Autodesk Inventor part; units mm, degrees
ref_plane "YZ Plane" through (0, 0, 0) normal (1, 0, 0) x (0, 1, 0)
ref_plane "XZ Plane" through (0, 0, 0) normal (0, 1, 0) x (-1, 0, 0)
ref_plane "XY Plane" through (0, 0, 0) normal (0, 0, 1) x (1, 0, 0)
sketch "Sketch1" plane through (0, 0, 0) normal (0, 0, 1) x (1, 0, 0)
  line L0 (0, 0) -> (50.8, 0)
  line L1 (50.8, 0) -> (50.8, 50.8)
  line L2 (50.8, 50.8) -> (0, 50.8)
  line L3 (0, 50.8) -> (0, 0)
  line L4 (1.5875, 49.2125) -> (49.2125, 49.2125)
  line L5 (49.2125, 49.2125) -> (49.2125, 1.5875)
  line L6 (49.2125, 1.5875) -> (1.5875, 1.5875)
  line L7 (1.5875, 1.5875) -> (1.5875, 49.2125)
  dimension "d0" = 50.8
  dimension "d1" = 50.8
  dimension "d2" = 1.5875
extrude "Extrusion1" add sketch "Sketch1" along normal blind 76.2
sketch "Sketch2" plane through (50.8, 0, 0) normal (1, 0, 0) x (0, 0, -1)
  circle A0 centre (-38.1, 25.4) radius 6.35
  line L0 (0, 0) -> (0, 50.8)
  line L1 (0, 50.8) -> (-76.2, 50.8)
  dimension "d5" = 12.7
  dimension "d16" = 38.1
  dimension "d17" = 25.4
extrude "Extrusion2" cut sketch "Sketch2" against normal blind 4.7625
sketch "Sketch3" plane through (0, 0, 0) normal (-1, 0, 0) x (0, 0, 1)
  circle A0 centre (38.1, 25.4) radius 6.35
  circle A1 centre (38.1, 25.4) radius 6.35
  point P0 (0, 0)
  dimension "d8" = 12.7
extrude "Extrusion3" cut sketch "Sketch3" against normal blind 4.7625
sketch "Sketch4" plane through (0, 0, 0) normal (-1, 0, 0) x (0, 0, 1)
  line L0 (0, 1.5875) -> (0, 49.2125) construction
  line L1 (0, 25.4) -> (12.7, 25.4) construction
  line L2 (12.7, 25.4) -> (63.5, 25.4) construction
  circle A0 centre (12.7, 25.4) radius 2.5797
  circle A1 centre (63.5, 25.4) radius 2.5797
  point P0 (0, 0)
  dimension "d11" = 12.7
  dimension "d12" = 50.8
  dimension "d13" = 5.1594
extrude "Extrusion4" cut sketch "Sketch4" against normal blind 55.5625
properties part number "new piston mount v2"
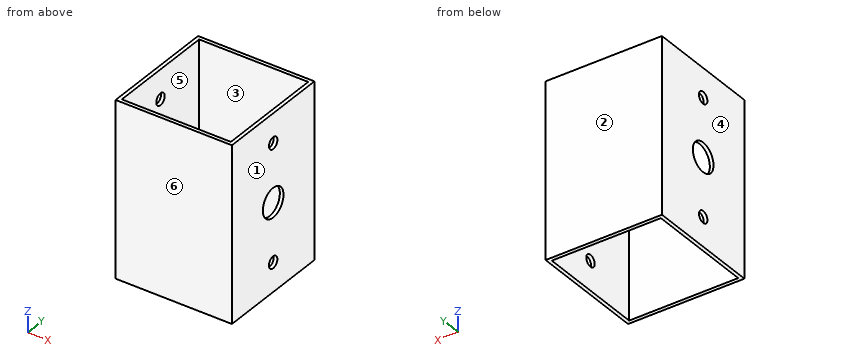
Design review of the part built by this model. Coordinates are the model's own, in mm. Face numbers are marked on the shaded views. A direction names the side the tool comes from. Coordinates: 2 decimals unless noted, no trailing zeros. Order: outer loops, then holes, each group sorted by start corner. A loop starts at its lowest first (then second) coordinate and runs counter-clockwise, first axis right, second up. Notation, with made-up numbers: M 17.5,-27 L 26.5,-27 A13 cw 26.5,-2 Z; hole C 74,20 d2. An arc over 180 degrees is marked long. Use a Markdown table: item, result.
(1) Add section C-C (y = 38.5). Give the boundary of the cut face in (x, z), then the cut area to 3 significant figures.
Worked answers:
| item | result |
|---|---|
| outline | M 0,0 L 1.59,0 L 1.59,76.2 L 0,76.2 Z; M 49.21,0 L 50.8,0 L 50.8,76.2 L 49.21,76.2 Z |
| area | 242 mm2 |
(2) For the marked faces 5 and 6, list the 3-axis set-ups (+Z, -Z, +X, -X, +Y, -Y) from which the entire face can be reached by the end or side of a thin tool; tool diameter is ignored.
Worked answers:
| item | result |
|---|---|
| face 5 | +Z, -Z |
| face 6 | +Z, -Z, +X, -X, -Y |
(3) Wall thickness on probe 1 along X at (y, z) = (27, 18.5); probe 2 along Y at (x, z) = (0.6, 63.5): over which ranges is each line inside the solid? List them lowest first.
Worked answers:
| item | result |
|---|---|
| probe 1 | x = 0 to 1.59, 49.21 to 50.8 |
| probe 2 | y = 0 to 22.82, 27.98 to 50.8 |
(4) Add section B-B (z = 63.5). Give the boundary of the cut face in (x, y).
Worked answers:
| item | result |
|---|---|
| outline | M 0,0 L 50.8,0 L 50.8,22.82 L 49.21,22.82 L 49.21,1.59 L 1.59,1.59 L 1.59,22.82 L 0,22.82 Z; M 0,27.98 L 1.59,27.98 L 1.59,49.21 L 49.21,49.21 L 49.21,27.98 L 50.8,27.98 L 50.8,50.8 L 0,50.8 Z |
(5) Draft analysis for pull direction X (two halves, no side actions). For the marked faces 1, 2, 3 and 4, state which applies: released by +X, released by -X, zero draft, split by the parting line, or undercut.
Worked answers:
| item | result |
|---|---|
| face 1 | released by +X |
| face 2 | zero draft |
| face 3 | undercut |
| face 4 | released by -X |
(6) Add section A-A (y = 25.4). Count the separate pieces of the cut face and the enclosed holes in it, then the cut area to 3 significant figures.
Worked answers:
| item | result |
|---|---|
| separate pieces | 8 |
| enclosed holes | 0 |
| area | 169 mm2 |
